Input: part model. Units: mm. Frame: model coordinates. A direction names the side the tool comes from. Coordinates: 2 decimals unless noted, no trailing zeros. Use one line per item in the form item = value. Start each with the question number.
(1) Set-up query: faces 5 (the face through (845.834, 4.88, -476.028)), 6 (the face through (424, 10, -507.888)). Return all of +Z, -Z, +X, -X, +Y, -Y with unobstructed straight access to the full face (end or side cutting, diameter ignored); none if empty.
(2) Pull-direction query (X, two-part tool) for faces 1 (the face through (-12.047, 4.88, 14.431)), 2 (the face through (866.1, 9.246, 18.7)), 3 (the face through (424, 10, 52.112)), 4 (the face through (-20, 10, -224)); classes: released by +X, released by -X, zero draft, split by the parting line, or undercut.
(3) Ray query, line 1 along X through (y, z) = (12, 26). Return the intervals inside material, ascending.
(4) First-contact query: pin 1 (15.5 mm diameter, centred on x = 0, z = -477.89, fed in from -Y); pin 2 (23 mm diameter, centred on x = 860.5, z = -475, fed in from -Y). Flat tips, straight axial feed; report the tip coordinate or a pass-through.
```python
from build123d import *

# Parameters (mm, degrees)
SKETCH1_W                                = 900
SKETCH1_H                                = 560
BOSS_EXTRUDE1_DEPTH                      = 20
CBORE_FOR_1_2_HEAVY_HEX_BOLT1_AT_2_COUNT = 2
CBORE_FOR_1_2_HEAVY_HEX_BOLT1_AT_2_PITCH = 860
CBORE_FOR_1_2_HEAVY_HEX_BOLT1_AT_3_COUNT = 2
CBORE_FOR_1_2_HEAVY_HEX_BOLT1_AT_3_PITCH = 994.786409236
CBORE_FOR_1_2_HEAVY_HEX_BOLT1_AT_4_COUNT = 2
CBORE_FOR_1_2_HEAVY_HEX_BOLT1_AT_4_PITCH = 500


with BuildPart() as part:
    # Sketch1 → Boss-Extrude1 (new body)
    with BuildSketch(Plane(origin=(0, 0, 0), x_dir=(1, 0, 0), z_dir=(0, 1, 0))):
        with Locations((430, 227.887771015)):
            Rectangle(SKETCH1_W, SKETCH1_H)
    extrude(amount=BOSS_EXTRUDE1_DEPTH)

    # Sketch3 → CBORE for 1/2 Heavy Hex Bolt1 (revolve, cut)
    with BuildSketch(Plane(origin=(0, 0, -477.887771015), x_dir=(0, 0, -1), z_dir=(1, 0, 0))):
        Polygon((0, 0), (0, 20), (6.74624, 20), (6.74624, 9.2456), (14.2875, 9.2456), (14.2875, 0.635), (14.9225, 0), align=None)
    cbore_for_1_2_heavy_hex_bolt1 = revolve(axis=Axis((0, -6.35, -477.887771015), (0, 1, 0)), mode=Mode.SUBTRACT)

    # CBORE for 1/2 Heavy Hex Bolt1 at 2: CBORE for 1/2 Heavy Hex Bolt1 ×2
    with Locations(*[(i * CBORE_FOR_1_2_HEAVY_HEX_BOLT1_AT_2_PITCH, 0, 0) for i in range(1, CBORE_FOR_1_2_HEAVY_HEX_BOLT1_AT_2_COUNT)]):
        add(cbore_for_1_2_heavy_hex_bolt1, mode=Mode.SUBTRACT)

    # CBORE for 1/2 Heavy Hex Bolt1 at 3: CBORE for 1/2 Heavy Hex Bolt1 ×2
    with Locations(*[Vector(0.864507187, 0, 0.502620457) * (i * CBORE_FOR_1_2_HEAVY_HEX_BOLT1_AT_3_PITCH) for i in range(1, CBORE_FOR_1_2_HEAVY_HEX_BOLT1_AT_3_COUNT)]):
        add(cbore_for_1_2_heavy_hex_bolt1, mode=Mode.SUBTRACT)

    # CBORE for 1/2 Heavy Hex Bolt1 at 4: CBORE for 1/2 Heavy Hex Bolt1 ×2
    with Locations(*[(0, 0, i * CBORE_FOR_1_2_HEAVY_HEX_BOLT1_AT_4_PITCH) for i in range(1, CBORE_FOR_1_2_HEAVY_HEX_BOLT1_AT_4_COUNT)]):
        add(cbore_for_1_2_heavy_hex_bolt1, mode=Mode.SUBTRACT)


solid = part.part
```
Values:
q1.face_5 = -Y
q1.face_6 = -Z, +X, -X, +Y, -Y
q2.face_1 = undercut
q2.face_2 = undercut
q2.face_3 = zero draft
q2.face_4 = released by -X
q3.line_1 = -20 to -5.51, 5.51 to 854.49, 865.51 to 880
q4.pin_1 = 9.25
q4.pin_2 = 0.49
